from build123d import *

# Parameters (mm, degrees)
F4_T = -2.54


with BuildPart() as f3:
    # F2 (on offset) → F3 section 0
    with BuildSketch(Plane.XY.offset(76.2)):
        Polygon((0, -25.4), (14.9297454082, -20.5490316571), (24.1568355139, -7.8490316571), (24.1568355139, 7.8490316571), (14.9297454082, 20.5490316571), (0, 25.4), (-14.9297454082, 20.5490316571), (-24.1568355139, 7.8490316571), (-24.1568355139, -7.8490316571), (-14.9297454082, -20.5490316571), align=None)
    # F0 (on Top) → F3 section 1
    with BuildSketch(Plane.XY):
        Polygon((-12.2329573114, -37.6491713284), (12.2329573114, -37.6491713284), (32.0262980243, -23.2684675292), (39.5866814257, 0), (32.0262980243, 23.2684675292), (12.2329573114, 37.6491713284), (-12.2329573114, 37.6491713284), (-32.0262980243, 23.2684675292), (-39.5866814257, 0), (-32.0262980243, -23.2684675292), align=None)
    loft()

    # F4
    f4_openings = [f3.faces().sort_by_distance(p)[0] for p in [
        (0, 0, 0),
    ]]
    offset(amount=F4_T, openings=f4_openings)


solid = f3.part
The listing builds one solid part. Answer for the finished solid, in the listing's coordinates (mm). Coordinates: 2 decimals unless noted, no trailing zeros. Answer in a Markdown table with one row per item. Add a question column.
1. Determine the mould class of faces 1 (the flat face through (0, 0, 73.66)), 2 (the flat face through (0, 0, 76.2)) for opening direction Y: +Y half, -Y half, draft (parallel to the pull), parting line (faces both ways), or undercut.
2. Consider line 1 (X direction, y = -33, z = 9); line 2 (X direction, y = -21, z = 30); line 3 (Y direction, x = -5, z = 22). Determine where each line is inside the solid, lowest interval first. Write a range as [from, to].
3. Flat-ended cylindrical pins translate along their axes: P1, Ø8, axis at x = 8.5, z = 37.5, coming from the -Y side; P2, Ø1, axis at x = 5.5, z = 22.5, coming from the -Y side; P3, Ø4, axis at x = -26.5, z = 39.5, coming from the +Y side. Find the tip coordinate at first contact, or state that the pin passes through.
Answer below:
| question | item | result |
|---|---|---|
| 1 | face 1 | undercut |
| 1 | face 2 | draft |
| 2 | line 1 | [-15.43, -10.85], [11.76, 15.99] |
| 2 | line 2 | [-25.81, -22.28], [20.68, 24.6] |
| 2 | line 3 | [-33.87, -31.3], [30.64, 33.23] |
| 3 | P1 | y = -30.76 |
| 3 | P2 | y = -33.2 |
| 3 | P3 | y = 18.61 |
